from build123d import *

# Parameters (mm, degrees)
EXTRUDE_START        = 79.5
SKETCH_4_R           = 4
EXTRUDE_1_DEPTH      = 15.5
SKETCH_5_R           = 3.4
EXTRUDE_2_DEPTH      = 1.95
SKETCH_6_R           = 4
EXTRUDE_3_DEPTH      = 86.05
EXTRUDE_START_2      = 74.85
EXTRUDE_4_DEPTH      = 5
CHAMFER_1_SIZE       = 0.58
CHAMFER_2_SIZE       = 0.6
CUT_EXTRUDE_START    = 57.05
SKETCH_9_OUTSIDE_W   = 36.078
SKETCH_9_OUTSIDE_H   = 38.09
SKETCH_9_OUTSIDE_W_2 = 6.8
SKETCH_9_OUTSIDE_H_2 = 15.011106998
CUT_EXTRUDE_1_DEPTH  = 5


with BuildPart() as part:
    # 草图4 → 凸台-拉伸1 (new body)
    with BuildSketch(Plane.XY.offset(EXTRUDE_START)):
        Circle(SKETCH_4_R)
    extrude(amount=-EXTRUDE_1_DEPTH)

    # 草图5 → 凸台-拉伸2 (add)
    with BuildSketch(Plane(origin=(0, 0, 64), x_dir=(-1, 0, 0), z_dir=(0, 0, -1))):
        with Locations(Location((0, 0, 0), (0, 0, 180))):
            Circle(SKETCH_5_R)
    extrude(amount=EXTRUDE_2_DEPTH)

    # 草图6 → 凸台-拉伸3 (add)
    with BuildSketch(Plane(origin=(0, 0, 62.05), x_dir=(-1, 0, 0), z_dir=(0, 0, -1))):
        with Locations(Location((0, 0, 0), (0, 0, 180))):
            Circle(SKETCH_6_R)
    extrude(amount=EXTRUDE_3_DEPTH)

    # 草图7 → 凸台-拉伸4 (add)
    with BuildSketch(Plane.XY.offset(EXTRUDE_START_2)):
        Polygon((6.5, -3.75277675), (6.5, 3.75277675), (0, 7.505553499), (-6.5, 3.75277675), (-6.5, -3.75277675), (0, -7.505553499), align=None)
    extrude(amount=-EXTRUDE_4_DEPTH)

    # 草图8 → 切除-旋转1 (revolve, cut)
    with BuildSketch(Plane(origin=(0, 0, 0), x_dir=(1, 0, 0), z_dir=(0, 1, 0))):
        Polygon((-6.5, -74.85), (-15.368693549, -74.85), (-15.368693549, -69.85), (-6.5, -69.85), (-13.368693549, -72.35), align=None)
    revolve(axis=Axis((0, 0, 52.5), (0, 0, 1)), mode=Mode.SUBTRACT)

    # 倒角1
    chamfer_1_edges = [part.edges().sort_by_distance(p)[0] for p in [
        (-4, 0, 79.5),
    ]]
    chamfer(chamfer_1_edges, length=CHAMFER_1_SIZE)

    # 倒角2
    chamfer_2_edges = [part.edges().sort_by_distance(p)[0] for p in [
        (-4, 0, 62.05),
    ]]
    chamfer(chamfer_2_edges, length=CHAMFER_2_SIZE - 0.0001)  # a hair under: the kernel refuses the full size

    # 草图9 outside → 切除-拉伸1 (cut)
    with BuildSketch(Plane.XY.offset(CUT_EXTRUDE_START)):
        Rectangle(SKETCH_9_OUTSIDE_W, SKETCH_9_OUTSIDE_H)
        Rectangle(SKETCH_9_OUTSIDE_W_2, SKETCH_9_OUTSIDE_H_2, mode=Mode.SUBTRACT)
    extrude(amount=CUT_EXTRUDE_1_DEPTH, mode=Mode.SUBTRACT)


solid = part.part
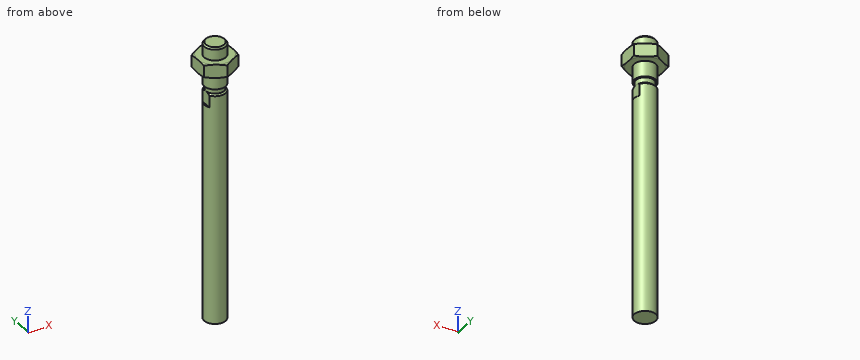
Here's how the part is built. I have some questions about the finished solid (model axes, mm). Round coordinates to 2 decimals unless told otherwise and drop trailing zeros. Loops run counter-clockwise (first coordinate to the right, second up) from the corner with the lowest first, then second, coordinate; pieces in that order, holes last. Notation, with made-up numbers: M 9,-1.5 L 65,-1.5 A34 cw 65,36.5 Z; hole C 45,47 d7. An arc over 180 degrees is marked long. Write each question's results on one line, items separated by ' | '. Start each with the question number.
(1) Will these pins go through, and if not, where does the flat tip stop? P1, Ø8, axis at y = -2, z = 62.5, coming from the +X side; P2, Ø6, axis at y = -3.5, z = 48, coming from the -X side; P3, Ø2, axis at y = 0, z = 59.5, coming from the +X side.
(2) If I drill on probe 1 along Z at (x, y) = (-0.25, 4.25); probe 2 along Z at (x, y) = (-1, -3.5); probe 3 along Z at (x, y) = (-0.5, 6.5), over which ranges is the centre line in solid material (lowest first)? Write a range as from..to.
(3) I want a section at A-A (z = -18). Please give me the cut outline in (x, y), then the cut area to 3 significant figures.
Solved:
1) P1: stops at x = 4 | P2: stops at x = -3.97 | P3: stops at x = 3.4
2) probe 1: z = 69.85..74.85 | probe 2: z = -24..61.81, 64..79.28 | probe 3: z = 69.86..74.84
3) outline: C 0,0 d8 | area: 50.3 mm²
